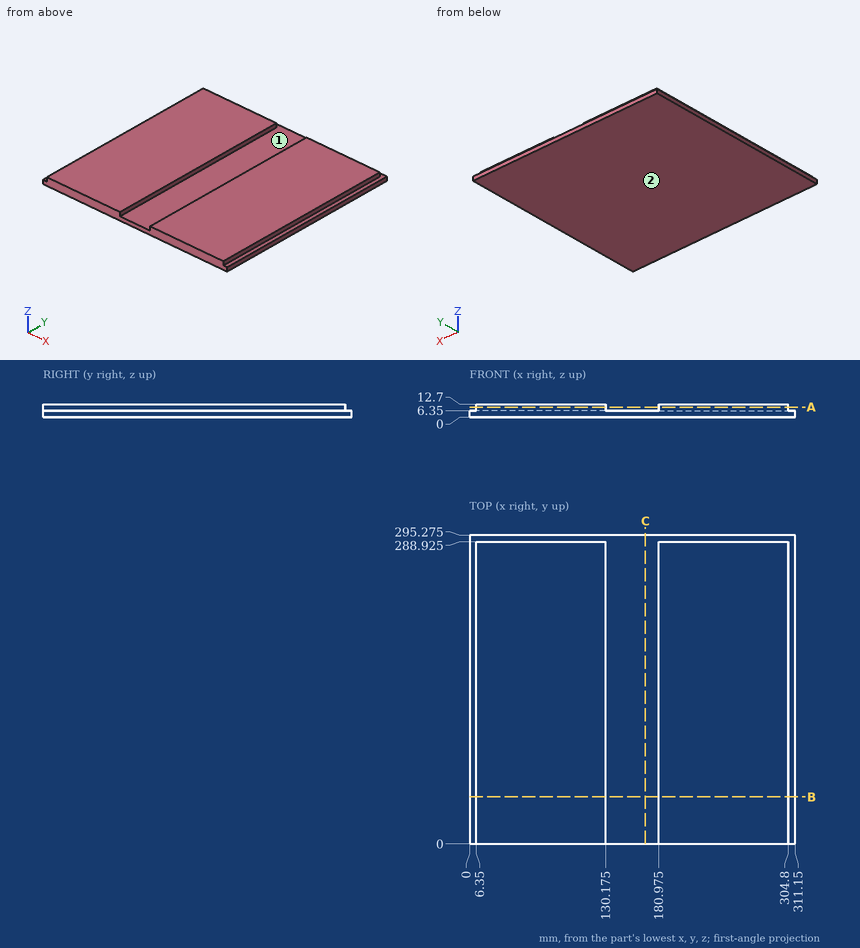
Drawing for the job (mm, zero at the part's lowest x, y, z). Give positions to 0.01 mm unless a question says otherwise; leave off trailing zeros. Write each loop counter-clockwise with the first axis right and the second up, starting at its lowest first coordinate (ties: lowest second). Pieces come first, ordered by that corner, then holes. Notation, with made-up numbers: (45.25, 14.5) -> (98.25, 14.5) arc R36 ccw to (98.25, 48.5) -> close; hole circle Ø2 at (-32, -11.5). An arc over 180 degrees is marked (long way). Put each result on its own line as item: value. Start each with the question number.
Item 1: Wall check: L1, parallel to X at y = 194, z = 11.5 (3 decimals); L2, parallel to Y at x = 286.5, z = 9.75 (3 decimals). Give the ranges that are in metal, low to high. Write a range as [from, to].
Item 2: Cut at B-B (y = 45). List the corners of the cut face in (x, z) (3 decimals).
Item 3: Pull direction X, two halves, no side cores. Call the marked faces 1 and 2: pulls with the +X half, pulls with the -X half, needs draft (parallel to the pull), parting line crosses it, or undercut.
Item 4: Pin check, flat tips, straight feed: pin 1 Ø5 at (x, z) = (76, 9) entering from +Y (3 decimals); pin 2 Ø5 at (y, z) = (134.5, 10) entering from -X. Stop position of each tip, or through.
Item 5: Cut at A-A (z = 9.75). List the corners of the cut face in (x, y) (3 decimals).
Item 6: Cut at C-C (x = 168). List the corners of the cut face in (y, z) (3 decimals).
Answer list:
1. L1: x = [6.35, 130.175], [180.975, 304.8]
1. L2: y = [0, 288.925]
2. outline: (0, 0) -> (311.15, 0) -> (311.15, 6.35) -> (304.8, 6.35) -> (304.8, 12.7) -> (180.975, 12.7) -> (180.975, 6.35) -> (130.175, 6.35) -> (130.175, 12.7) -> (6.35, 12.7) -> (6.35, 6.35) -> (0, 6.35) -> close
3. face 1: undercut
3. face 2: needs draft
4. pin 1: stops at y = 288.925
4. pin 2: stops at x = 6.35
5. outline: (6.35, 0) -> (130.175, 0) -> (130.175, 288.925) -> (6.35, 288.925) -> close; (180.975, 0) -> (304.8, 0) -> (304.8, 288.925) -> (180.975, 288.925) -> close
6. outline: (0, 0) -> (295.275, 0) -> (295.275, 6.35) -> (0, 6.35) -> close
